Could you check a few things on this drawing? It's one solid part, dimensions in mm from its lowest x, y, z. Give positions to 0.01 mm unless a question says otherwise; leave off trailing zeros. Loops run counter-clockwise (first coordinate to the right, second up) from the corner with the lowest first, then second, coordinate; pieces in that order, holes last. Notation, with made-up numbers: (38, 57) - (64, 57) arc R26 cw to (64, 84) - close; hole circle Ø1 at (-23.75, 16). An arc over 180 degrees is marked (long way). Return JSON: item names as keys, results as strings. Group by question number.
(1) For P1, Ø8, axis at x = 195.5, z = 26.5, coming from the -Y side; P2, Ø1.5, axis at x = 209, y = 343.5, coming from the +Z side (1 decimal); P3, Ø1, axis at y = 69, z = 37.5, coming from the +X side (1 decimal), each with a flat end and sliding along its axis, tell me the tip position at first contact or that it passes through.
(2) If we section it at D-D (y = 26.5): Please give me the cut outline in (x, z) (1 decimal).
(3) If we section it at C-C (y = 299.75): Please give me the cut outline in (x, z) (1 decimal).
(4) If we mould it in two halves opening along Y, with no side actions, what happens to the marked faces 1, 2 and 3? For each: released by +Y, released by -Y, zero draft, split by the parting line, or undercut.
(5) If we section it at A-A (z = 13): State how many separate pieces and enclosed holes the cut face has, then the cut area to 3 significant figures.
(6) I need wall thicknesses on probe 1 along Y at (x, z) = (125, 15); probe 2 along Z at (x, y) = (107, 155) (1 decimal); probe 3 along Y at (x, z) = (98, 27). Which ranges of each line are inside material? Lowest first, please. Write a range as [from, to].
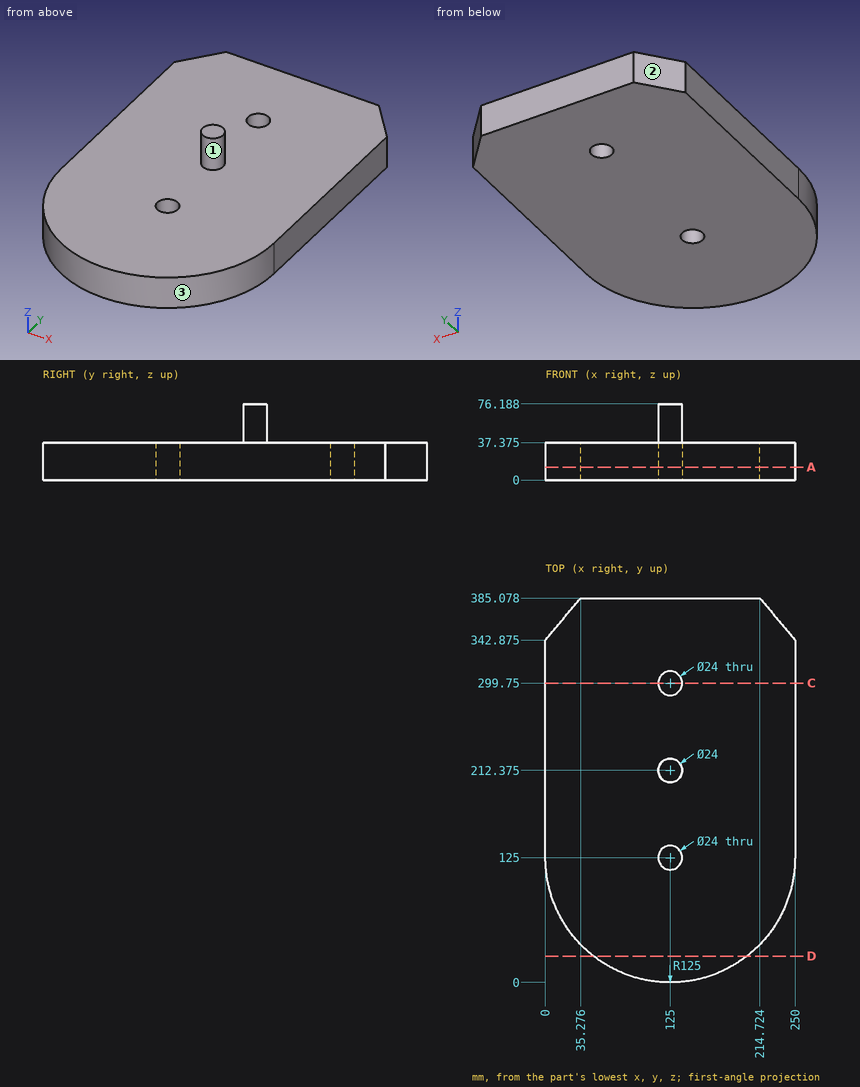
Values:
{
 "1": {"P1": "y = 19.16", "P2": "z = 37.4", "P3": "x = 237"},
 "2": {"outline": "(48, 0) - (202, 0) - (202, 37.4) - (48, 37.4) - close"},
 "3": {"outline": "(0, 0) - (113, 0) - (113, 37.4) - (0, 37.4) - close; (137, 0) - (250, 0) - (250, 37.4) - (137, 37.4) - close"},
 "4": {"face 1": "split by the parting line", "face 2": "released by +Y", "face 3": "released by -Y"},
 "5": {"separate pieces": "1", "enclosed holes": "2", "area": "87,200 mm2"},
 "6": {"probe 1": "[0, 113], [137, 287.75], [311.75, 385.08]", "probe 2": "[0, 37.4]", "probe 3": "[2.95, 385.08]"}
}
